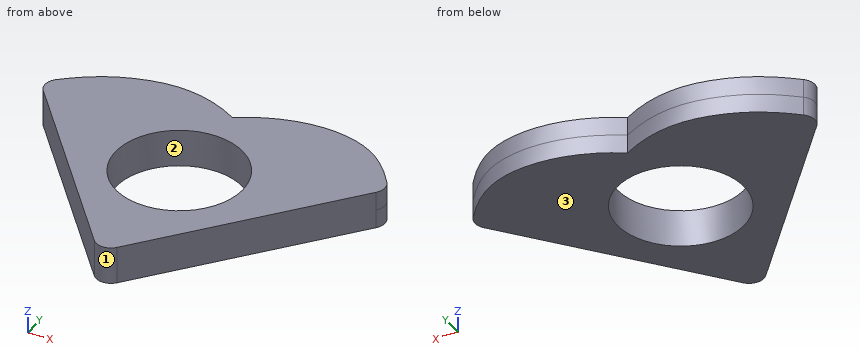
from build123d import *

# Parameters (mm, degrees)
F1_DEPTH = 2.5
F2_R     = 8.5
F3_DEPTH = 5
F4_R     = 2


with BuildPart() as f1:
    # F0 (on Top) → F1 (new body, symmetric)
    with BuildSketch(Plane.XY):
        with BuildLine():
            add(Edge.make_bspline(
                [(0, 12.8306830302), (-5.6033253596, 16.1092708646), (-14.1634437691, 15.2185435642), (-19.7434784059, 11.930183225), (-23.3991518617, 8.4396265447)],
                knots=[0, 0, 0, 0, 0.5245675833, 1, 1, 1, 1], degree=3))
            Line((-23.3991518617, 8.4396265447), (0, -19.5570103824))
            Line((0, -19.5570103824), (23.3991537243, 8.4396265447))
            add(Edge.make_bspline(
                [(23.3991537243, 8.4396265447), (21.1730352272, 11.6721171587), (16.5383048632, 17.0813520932), (5.7577232004, 16.5454135329), (0, 12.8306830302)],
                knots=[0, 0, 0, 0, 0.4436460764, 1, 1, 1, 1], degree=3))
        make_face()
    extrude(amount=F1_DEPTH, both=True)

    # F2 (on face) → F3 (cut)
    with BuildSketch(Plane.XY.offset(2.5)):
        Circle(F2_R)
    extrude(amount=-F3_DEPTH, mode=Mode.SUBTRACT)

    # F4
    f4_edges = [f1.edges().sort_by_distance(p)[0] for p in [
        (-23.399152, 8.439627, -1.25),
        (-23.399152, 8.439627, 1.25),
        (23.399154, 8.439627, -1.25),
        (23.399154, 8.439627, 1.25),
        (0, -19.55701, 0),
    ]]
    fillet(f4_edges, radius=F4_R)


solid = f1.part
Check sheet for the modelled part. Datum: model origin and axes. Units: mm. Face numbers are marked on the shaded views. Give positions to 0.01 mm unless a question says otherwise; leave off trailing zeros. Loops run counter-clockwise (first coordinate to the right, second up) from the corner with the lowest first, then second, coordinate; pieces in that order, holes last. Notation, with made-up numbers: M 43.25,13.5 L 100.25,13.5 A28 ccw 100.25,48.5 Z; hole C -28.5,-16 d1. An arc over 180 degrees is marked long. Use a Markdown table: item, result. Add a question column.
Q1. Scan lines: line 1 along X through (y, z) = (0.5, 0.2); line 2 along X through (y, z) = (-3, 0.2); line 3 along Y through (x, z) = (0, -0.85). Record each from-to range of solid material in increasing order. Write a range as [from, to].
Q2. Sectioned sample at B-B, the plane y = 0. Record the cut outline in (x, z).
Q3. Go/stop test with flat-tipped pins: pin 1 (3 mm diameter, centred on y = 4, z = 1.5, fed in from +X); pin 2 (10 mm diameter, centred on x = 0, y = 0, fed in from -Z). Record where each tip stops, or that it passes through.
Q4. Sectioned sample at A-A, the plane y = -7. Record the cut outline in (x, z).
Q5. Mould release check, pull along X, two halves, no side actions. Record for the marked faces 1, 2 and 3: pulls with the +X half, pulls with the -X half, needs draft (parallel to the pull), parting line crosses it, or undercut.
Verdict:
| question | item | result |
|---|---|---|
| 1 | line 1 | [-16.76, -8.49], [8.49, 16.76] |
| 1 | line 2 | [-13.84, -7.95], [7.95, 13.84] |
| 1 | line 3 | [-18.44, -8.5], [8.5, 12.83] |
| 2 | outline | M -16.35,-2.5 L -8.5,-2.5 L -8.5,2.5 L -16.35,2.5 Z; M 8.5,-2.5 L 16.35,-2.5 L 16.35,2.5 L 8.5,2.5 Z |
| 3 | pin 1 | x = 20.94 |
| 3 | pin 2 | through |
| 4 | outline | M -10.49,-2.5 L -4.82,-2.5 L -4.82,2.5 L -10.49,2.5 Z; M 4.82,-2.5 L 10.49,-2.5 L 10.49,2.5 L 4.82,2.5 Z |
| 5 | face 1 | parting line crosses it |
| 5 | face 2 | undercut |
| 5 | face 3 | needs draft |
